```python
from build123d import *

# Parameters (mm, degrees)
SALIENTE_EXTRUIR1_DEPTH = 7
CROQUIS2_W              = 3.5
CROQUIS2_H              = 4
SALIENTE_EXTRUIR2_DEPTH = 4
CROQUIS3_W              = 11.5
CROQUIS3_H              = 5
SALIENTE_EXTRUIR3_DEPTH = 3
SALIENTE_EXTRUIR4_START = -7
CROQUIS4_W              = 4.5
CROQUIS4_H              = 5
SALIENTE_EXTRUIR4_DEPTH = 11
REDONDEO3_R             = 2


with BuildPart() as part:
    # Croquis1 → Saliente-Extruir1 (new, symmetric)
    with BuildSketch(Plane.XY):
        with BuildLine():
            Line((-12, -10.5), (12, -10.5))
            Line((12, -10.5), (12, 10.33406025))
            Line((12, 10.33406025), (0.5, 10.33406025))
            Line((0.5, 10.33406025), (0.5, 7.83406025))
            ThreePointArc((0.5, 7.83406025), (4.342612549, 6.539435468), (7.026556767, 3.5))
            Line((7.026556767, 3.5), (9.15, 3.5))
            Line((9.15, 3.5), (9.15, -3.5))
            Line((9.15, -3.5), (7.026556767, -3.5))
            ThreePointArc((7.026556767, -3.5), (-6.539435468, -4.342612549), (-0.5, 7.83406025))
            Line((-0.5, 7.83406025), (-0.5, 10.33406025))
            Line((-0.5, 10.33406025), (-12, 10.33406025))
            Line((-12, 10.33406025), (-12, -10.5))
        make_face()
    extrude(amount=SALIENTE_EXTRUIR1_DEPTH, both=True)

    # Croquis2 → Saliente-Extruir2 (add)
    with BuildSketch(Plane.XY.offset(-7)):
        with Locations((2.25, 12.33406025)):
            Rectangle(CROQUIS2_W, CROQUIS2_H)
        with Locations((-2.25, 12.33406025)):
            Rectangle(CROQUIS2_W, CROQUIS2_H)
    extrude(amount=SALIENTE_EXTRUIR2_DEPTH)

    # Croquis3 → Saliente-Extruir3 (add)
    with BuildSketch(Plane(origin=(0, 0, 7), x_dir=(-1, 0, 0), z_dir=(0, 0, -1))):
        with Locations((-6.25, 12.83406025)):
            Rectangle(CROQUIS3_W, CROQUIS3_H)
        with Locations((6.25, 12.83406025)):
            Rectangle(CROQUIS3_W, CROQUIS3_H)
    extrude(amount=SALIENTE_EXTRUIR3_DEPTH)

    # Croquis4 → Saliente-Extruir4 (add)
    with BuildSketch(Plane.XY.offset(SALIENTE_EXTRUIR4_START)):
        with Locations((-9.75, 12.83406025)):
            Rectangle(CROQUIS4_W, CROQUIS4_H)
        with Locations((9.75, 12.83406025)):
            Rectangle(CROQUIS4_W, CROQUIS4_H)
    extrude(amount=SALIENTE_EXTRUIR4_DEPTH)

    # Redondeo3
    redondeo3_edges = [part.edges().sort_by_distance(p)[0] for p in [
        (12, -10.5, 0),
        (-12, -10.5, 0),
        (12, 15.33406025, 0),
        (-12, 15.33406025, 0),
    ]]
    fillet(redondeo3_edges, radius=REDONDEO3_R)


solid = part.part
```
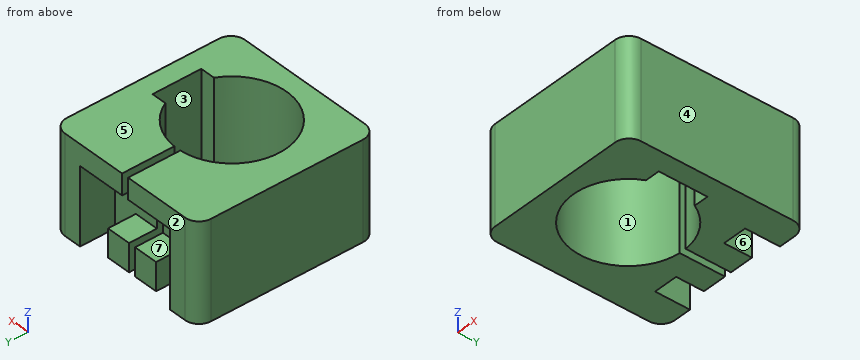
Source: CAD feature listing. Evaluate the final solid. Frame: model axes, mm. Face numbers are marked on the shaded views. A direction names the side the tool comes from. Give positions to 0.01 mm unless a question says otherwise; leave off trailing zeros. Loops run counter-clockwise (first coordinate to the right, second up) from the corner with the lowest first, then second, coordinate; pieces in that order, holes last. Notation, with made-up numbers: (-3, 65.5) -> (20, 65.5) arc R14 ccw to (20, 82.5) -> close; hole circle Ø6 at (69, 6.5). An arc over 180 degrees is marked (long way). Use a Markdown table: item, result. Add a question column.
(1) Pull-direction query (Y, two-part tool) for the marked faces 1, 2, 3 and 4; classes: +Y half, -Y half, draft (parallel to the pull), parting line (faces both ways), or undercut.
(2) Section query B-B (z = 0.5). Output: boundary loops of the cut face in (x, y).
(3) Ray query, line 1 (X direction, y = 0, z = 0); line 2 (X direction, y = 10, z = 6); line 3 (Y direction, x = -6.75, z = 5.75). Return the intervals inside material, ascending.
(4) Section query C-C (x = 5.75). Output: boundary loops of the cut face in (y, z).
(5) Section query A-A (y = 0). Output: boundary loops of the cut face in (x, z).
(6) Section query D-D (y = 11). Output: boundary loops of the cut face in (x, z).
(7) First-contact query: pin 1 Ø1 at (x, z) = (-3, -6) entering from +Y; pin 2 Ø7.5 at (x, z) = (-4, -3) entering from +Y; pin 3 Ø2.5 at (x, y) = (-5.5, 12.5) entering from -Z. Flat tips, straight axial feed; report the tip coordinate or a pass-through.
(8) Access query for the marked faces 5, 6 and 7. Directions: +Z, -Z, +X, -X, +Y, -Y. A direction counts if a zero-diameter tool reaches every point of the face in a straight line with its end or side. Return the directions, or none.
Checked values:
| question | item | result |
|---|---|---|
| 1 | face 1 | undercut |
| 1 | face 2 | +Y half |
| 1 | face 3 | undercut |
| 1 | face 4 | draft |
| 2 | outline | (-12, -8.5) arc R2 ccw to (-10, -10.5) -> (10, -10.5) arc R2 ccw to (12, -8.5) -> (12, 13.33) arc R2 ccw to (10, 15.33) -> (7.5, 15.33) -> (7.5, 10.33) -> (0.5, 10.33) -> (0.5, 7.83) arc R7.85 cw to (7.03, 3.5) -> (9.15, 3.5) -> (9.15, -3.5) -> (7.03, -3.5) arc R7.85 cw (long way) to (-0.5, 7.83) -> (-0.5, 10.33) -> (-7.5, 10.33) -> (-7.5, 15.33) -> (-10, 15.33) arc R2 ccw to (-12, 13.33) -> close |
| 3 | line 1 | -12 to -7.85, 9.15 to 12 |
| 3 | line 2 | -12 to -0.5, 0.5 to 12 |
| 3 | line 3 | -10.5 to -4.01, 4.01 to 15.33 |
| 4 | outline | (-10.5, -7) -> (-5.34, -7) -> (-5.34, 7) -> (-10.5, 7) -> close; (5.34, -7) -> (10.33, -7) -> (10.33, 4) -> (15.33, 4) -> (15.33, 7) -> (5.34, 7) -> close |
| 5 | outline | (-12, -7) -> (-7.85, -7) -> (-7.85, 7) -> (-12, 7) -> close; (9.15, -7) -> (12, -7) -> (12, 7) -> (9.15, 7) -> close |
| 6 | outline | (-12, -7) -> (-7.5, -7) -> (-7.5, 4) -> (-0.5, 4) -> (-0.5, 7) -> (-12, 7) -> close; (-4, -7) -> (-0.5, -7) -> (-0.5, -3) -> (-4, -3) -> close; (0.5, -7) -> (4, -7) -> (4, -3) -> (0.5, -3) -> close; (0.5, 4) -> (7.5, 4) -> (7.5, -7) -> (12, -7) -> (12, 7) -> (0.5, 7) -> close |
| 7 | pin 1 | y = 14.33 |
| 7 | pin 2 | y = 15.33 |
| 7 | pin 3 | z = 4 |
| 8 | face 5 | +Z, +X, -X, +Y, -Y |
| 8 | face 6 | -Z, +Y |
| 8 | face 7 | +Y |
